Could you check a few things on this model? Use its own coordinates, in mm. Face numbers are marked on the shaded views. A direction names the side the tool comes from. Round coordinates to 2 decimals unless told otherwise and drop trailing zeros. Write each loop counter-clockwise with the first axis right and the second up, starting at its lowest first coordinate (ties: lowest second). Pieces come first, ordered by that corner, then holes. Notation, with made-up numbers: (77, 20.5) - (86, 20.5) arc R16 cw to (86, 27.5) - close; hole circle Ø7 at (-14, 46.5). An arc over 180 degrees is marked (long way). Put each result on its own line as item: value.
from build123d import *

# Parameters (mm, degrees)
F3_R = 2


with BuildPart() as f1:
    # F0 (on Front) → F1 (revolve)
    with BuildSketch(Plane.XZ):
        with BuildLine():
            Line((67.0871215252, 15.234352517), (0, 15.234352517))
            Line((0, 15.234352517), (0, 0.234352517))
            Line((0, 0.234352517), (125, 0.234352517))
            Line((125, 0.234352517), (125, 15.234352517))
            Line((125, 15.234352517), (95, 15.234352517))
            Line((95, 15.234352517), (95, 30.234352517))
            Line((95, 30.234352517), (90, 30.234352517))
            ThreePointArc((90, 30.234352517), (87.2613872125, 29.4176526497), (85.417424305, 27.234352517))
            ThreePointArc((85.417424305, 27.234352517), (78.0415726753, 18.5011519863), (67.0871215252, 15.234352517))
        make_face()
    revolve(axis=Axis((62.5, 0, 0.234352517), (-1, 0, 0)))

    # F2: F1 across face


with BuildPart() as f1_1:
    add(f1.part)
    add(f1.part.mirror(Plane(origin=(0, 0, 0.234352517), x_dir=(0, -1, 0), z_dir=(-1, 0, 0))))

    # F3
    f3_edges = [f1_1.edges().sort_by_distance(p)[0] for p in [
        (-125, 0, -14.765647),
        (125, 0, -14.765647),
    ]]
    fillet(f3_edges, radius=F3_R)


solid = f1_1.part
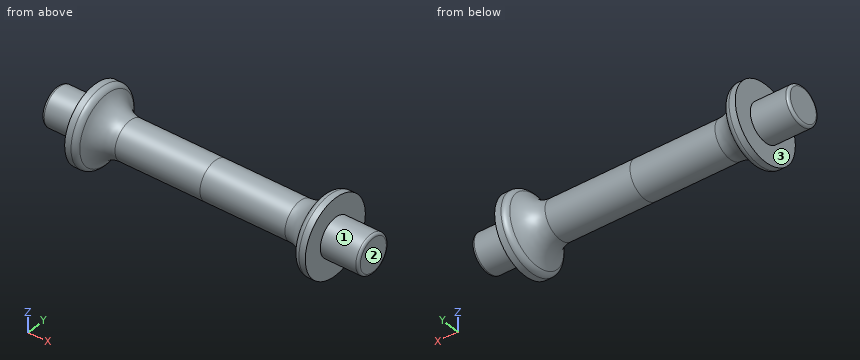
(1) Please list where these lines run through material, in increasing order: probe 1 along X at (y, z) = (-14, -13); probe 2 along X at (y, z) = (19.5, -4.5); probe 3 along Z at (x, y) = (16.5, 7). Write a range as from..to.
Values found:
probe 1: x = -95..-79.43, 79.43..95
probe 2: x = -95..-80.39, 80.39..95
probe 3: z = -13.03..13.5
(2) I'm going to push flat-ended pins straight in: pin 1 (8 mm diameter, centred on y = 22.5, z = 8.5, fed in from -X); pin 2 (3 mm diameter, centred on x = 88, y = 16, fed in from -Z); pin 3 (3 mm diameter, centred on x = -54.5, z = 11.5, fed in from +Y); pin 4 (18 mm diameter, centred on y = 5.5, z = 14.5, fed in from +X). Where does each tip first touch, or does it pass through?
Values found:
pin 1: stops at x = -95
pin 2: stops at z = -25.74
pin 3: stops at y = 11.39
pin 4: stops at x = 125
(3) Imagine slicing it at B-B, the plane x = -15. List the corners of the cut face in (y, z) for me.
Values found:
outline: circle Ø30 at (0, 0.23)
(4) Imagine slicing it at A-A, the plane y = 0. List the corners of the cut face in (x, z) for me, then the cut area to 3 significant figures.
Values found:
outline: (-125, -12.77) arc R2 ccw to (-123, -14.77) - (-95, -14.77) - (-95, -29.77) - (-90, -29.77) arc R5 ccw to (-85.42, -26.77) arc R20 cw to (-67.09, -14.77) - (67.09, -14.77) arc R20 cw to (85.42, -26.77) arc R5 ccw to (90, -29.77) - (95, -29.77) - (95, -14.77) - (123, -14.77) arc R2 ccw to (125, -12.77) - (125, 13.23) arc R2 ccw to (123, 15.23) - (95, 15.23) - (95, 30.23) - (90, 30.23) arc R5 ccw to (85.42, 27.23) arc R20 cw to (67.09, 15.23) - (-67.09, 15.23) arc R20 cw to (-85.42, 27.23) arc R5 ccw to (-90, 30.23) - (-95, 30.23) - (-95, 15.23) - (-123, 15.23) arc R2 ccw to (-125, 13.23) - close
area: 8,300 mm^2
(5) For the marked faces 1, 2 and 3, which set-ups out of +Z, -Z, +X, -X, +Y, -Y let a thin tool reach every point of the face, with its end or its side?
Values found:
face 1: +X
face 2: +Z, -Z, +X, +Y, -Y
face 3: -X
